The model under review builds one solid part; all positions refer to its coordinate system, in mm. A direction names the side the tool comes from. Coordinates: 2 decimals unless noted, no trailing zeros. Loops run counter-clockwise (first coordinate to the right, second up) from the corner with the lowest first, then second, coordinate; pieces in that order, holes last. Notation, with made-up numbers: M 84.25,69 L 136.25,69 A22 ccw 136.25,81 Z; hole C -25,-2.5 d7. An arc over 180 degrees is marked long. One line per item, written item: value.
```python
from build123d import *

# Parameters (mm, degrees)
CROQUIS1_R                     = 5
SALIENTE_EXTRUIR1_DEPTH        = 10
SALIENTE_EXTRUIR1_DEPTH_BACK   = 10
CROQUIS1_R_2                   = 4
SALIENTE_EXTRUIR1_2_DEPTH      = 10
SALIENTE_EXTRUIR1_2_DEPTH_BACK = 10
SALIENTE_EXTRUIR2_DEPTH        = 5


with BuildPart() as part:
    # Croquis1 → Saliente-Extruir1 (new body, two sides)
    with BuildSketch(Plane.XY) as saliente_extruir1_sk:
        with Locations((-30, 0)):
            Circle(CROQUIS1_R)
    extrude(amount=SALIENTE_EXTRUIR1_DEPTH)
    extrude(saliente_extruir1_sk.sketch, amount=-SALIENTE_EXTRUIR1_DEPTH_BACK)



with BuildPart() as body_2:
    # Croquis1 → Saliente-Extruir1 2 (new body, two sides)
    with BuildSketch(Plane.XY) as saliente_extruir1_2_sk:
        with Locations((30, 0)):
            Circle(CROQUIS1_R_2)
    extrude(amount=SALIENTE_EXTRUIR1_2_DEPTH)
    extrude(saliente_extruir1_2_sk.sketch, amount=-SALIENTE_EXTRUIR1_2_DEPTH_BACK)


with BuildPart() as part_1:
    add(part.part)

    add(body_2.part)  # Saliente-Extruir2 merges body 2
    # Croquis2 → Saliente-Extruir2 (add)
    with BuildSketch(Plane.XY.offset(10)):
        with BuildLine():
            Line((-30, 7), (30, 7))
            ThreePointArc((30, 7), (37, 0), (30, -7))
            Line((30, -7), (-30, -7))
            ThreePointArc((-30, -7), (-37, 0), (-30, 7))
        make_face()
    saliente_extruir2 = extrude(amount=SALIENTE_EXTRUIR2_DEPTH)

    # Simetr_a1: Saliente-Extruir2 across plane
    add(saliente_extruir2.mirror(Plane.XY))


solid = part_1.part
```
(1) Add section B-B on y = 0. State the section outline as (x, z) points.
Checks:
outline: M -37,-15 L 37,-15 L 37,-10 L 34,-10 L 34,10 L 37,10 L 37,15 L -37,15 L -37,10 L -35,10 L -35,-10 L -37,-10 Z; hole M -25,-10 L 26,-10 L 26,10 L -25,10 Z
(2) Add section A-A on x = -21. State the section outline as (y, z) points, then the cut area to 3 significant figures.
Checks:
outline: M -7,-15 L 7,-15 L 7,-10 L -7,-10 Z; M -7,10 L 7,10 L 7,15 L -7,15 Z
area: 140 mm^2
(3) Add section D-D on y = 5.75. State the section outline as (x, z) points.
Checks:
outline: M -33.99,-15 L 33.99,-15 L 33.99,-10 L -33.99,-10 Z; M -33.99,10 L 33.99,10 L 33.99,15 L -33.99,15 Z
(4) Draft analysis for pull direction X (two halves, no side actions). For faces 3 (the face through (0, -7, -12)), 4 (the face through (-37, 0, 12)), 5 (the face through (1, 0, -10)), state which applies: pulls with the +X half, pulls with the -X half, needs draft (parallel to the pull), parting line crosses it, or undercut.
Checks:
face 3: needs draft
face 4: pulls with the -X half
face 5: undercut
(5) Tool access review of faces 1 (the face through (-35, 0, 0)), 2 (the face through (37, 0, 12)): name each direction out of +Z, -Z, +X, -X, +Y, -Y from which nothing blocks a thin tool from reaching the whole face with its end or side.
Checks:
face 1: none
face 2: +Z, -Z, +X
(6) Insertion check: pin 1 Ø4 at (x, z) = (27.5, 5) entering from +Y; pin 2 Ø3 at (y, z) = (3.5, 9.5) entering from -X; pin 3 Ø8 at (y, z) = (-4.5, 9) entering from -X; pin 4 Ø8 at (x, z) = (-20, -3.5) entering from +Y. Each pin has a flat end and moves straight along its axis. Give the tip position at first contact, or say it passes through.
Checks:
pin 1: y = 3.97
pin 2: x = -36.68
pin 3: x = -36.97
pin 4: through
(7) To check wall thickness, follow L1, parallel to Z at x = 1, y = -4.5; L2, parallel to X at y = -0.25, z = 2; L3, parallel to X at y = 1.5, z = -1.25. State the ranges of each line that lie inside material, in increasing order. Write a range as [from, to].
Checks:
L1: [-15, -10], [10, 15]
L2: [-34.99, -25.01], [26.01, 33.99]
L3: [-34.77, -25.23], [26.29, 33.71]
(8) Add section C-C on z = 4.5. State the section outline as (x, y) points, then the cut area to 3 significant figures.
Checks:
outline: C -30,0 d10; C 30,0 d8
area: 129 mm^2
